The listing builds one solid part. Answer for the finished solid, in the listing's coordinates (mm). A direction names the side the tool comes from. Coordinates: 2 decimals unless noted, no trailing zeros. Write each loop counter-clockwise with the first axis right and the second up, starting at its lowest first coordinate (ties: lowest second). Pieces come first, ordered by that corner, then holes. Notation, with made-up numbers: M 55.5,37 L 101.5,37 A28 ccw 101.5,62 Z; hole C -3,43.5 d2. An arc over 180 degrees is marked long. Answer as CSV lines item,"result".
```python
from build123d import *

# Parameters (mm, degrees)
BOSS_EXTRUDE1_DEPTH = 1.57
SKETCH2_W           = 4.040944922
SKETCH2_H           = 4.040944922
BOSS_EXTRUDE2_DEPTH = 1.57


with BuildPart() as part:
    # Sketch1 → Boss-Extrude1 (new body)
    with BuildSketch(Plane.XY):
        with BuildLine():
            Line((10, 2), (10, 40))
            Line((10, 40), (0, 40))
            Line((0, 40), (0, 32))
            ThreePointArc((0, 32), (1.414213562, 31.414213562), (2, 30))
            ThreePointArc((2, 30), (1.414213562, 28.585786438), (0, 28))
            Line((0, 28), (0, 12.75))
            ThreePointArc((0, 12.75), (1.944543648, 11.944543648), (2.75, 10))
            ThreePointArc((2.75, 10), (1.944543648, 8.055456352), (0, 7.25))
            Line((0, 7.25), (0, 0))
            Line((0, 0), (8, 0))
            ThreePointArc((8, 0), (8.585786438, 1.414213562), (10, 2))
        make_face()
        with BuildLine():
            Line((20, 40), (10, 40))
            Line((10, 40), (10, 2))
            ThreePointArc((10, 2), (11.414213562, 1.414213562), (12, 0))
            Line((12, 0), (20, 0))
            Line((20, 0), (20, 7.25))
            ThreePointArc((20, 7.25), (17.25, 10), (20, 12.75))
            Line((20, 12.75), (20, 28))
            ThreePointArc((20, 28), (18, 30), (20, 32))
            Line((20, 32), (20, 40))
        make_face()
        with BuildLine():
            ThreePointArc((2, 30), (1.414213562, 31.414213562), (0, 32))
            Line((0, 32), (0, 31.11))
            ThreePointArc((0, 31.11), (0.784888527, 30.784888527), (1.11, 30))
            ThreePointArc((1.11, 30), (0.784888527, 29.215111473), (0, 28.89))
            Line((0, 28.89), (0, 28))
            ThreePointArc((0, 28), (1.414213562, 28.585786438), (2, 30))
        make_face()
        with BuildLine():
            Line((0, 31.11), (0, 32))
            ThreePointArc((0, 32), (-2, 30), (0, 28))
            Line((0, 28), (0, 28.89))
            ThreePointArc((0, 28.89), (-1.11, 30), (0, 31.11))
        make_face()
        with BuildLine():
            ThreePointArc((22, 30), (21.414213562, 31.414213562), (20, 32))
            Line((20, 32), (20, 31.11))
            ThreePointArc((20, 31.11), (20.784888527, 30.784888527), (21.11, 30))
            ThreePointArc((21.11, 30), (20.784888527, 29.215111473), (20, 28.89))
            Line((20, 28.89), (20, 28))
            ThreePointArc((20, 28), (21.414213562, 28.585786438), (22, 30))
        make_face()
        with BuildLine():
            Line((20, 31.11), (20, 32))
            ThreePointArc((20, 32), (18, 30), (20, 28))
            Line((20, 28), (20, 28.89))
            ThreePointArc((20, 28.89), (18.89, 30), (20, 31.11))
        make_face()
        with BuildLine():
            ThreePointArc((8, 0), (10, -2), (12, 0))
            Line((12, 0), (11.11, 0))
            ThreePointArc((11.11, 0), (10, -1.11), (8.89, 0))
            Line((8.89, 0), (8, 0))
        make_face()
        with BuildLine():
            ThreePointArc((12, 0), (11.414213562, 1.414213562), (10, 2))
            Line((10, 2), (10, 1.11))
            ThreePointArc((10, 1.11), (10.784888527, 0.784888527), (11.11, 0))
            Line((11.11, 0), (12, 0))
        make_face()
        with BuildLine():
            Line((10, 1.11), (10, 2))
            ThreePointArc((10, 2), (8.585786438, 1.414213562), (8, 0))
            Line((8, 0), (8.89, 0))
            ThreePointArc((8.89, 0), (9.215111473, 0.784888527), (10, 1.11))
        make_face()
    extrude(amount=BOSS_EXTRUDE1_DEPTH)

    # Sketch2 → Boss-Extrude2 (add)
    with BuildSketch(Plane(origin=(0, 0, 0), x_dir=(-1, 0, 0), z_dir=(0, 0, -1))):
        with Locations((-10, 10)):
            Rectangle(SKETCH2_W, SKETCH2_H)
    extrude(amount=BOSS_EXTRUDE2_DEPTH)


solid = part.part
```
Q1. For faces 1 (the flat face through (20, 20, 1)), 2 (the flat face through (0, 36, 1)), 3 (the flat face through (12.02, 10, -1)), 4 (the flat face through (20, 36, 1)), 5 (the flat face through (0, 20, 1)), determine the directions among +Z, -Z, +X, -X, +Y, -Y from which every point of the face is accessible in a straight line to the end or side of a thin tool.
Output:
face 1,"+Z, -Z, +X, -Y"
face 2,"+Z, -Z, -X, +Y"
face 3,"-Z, +X, +Y, -Y"
face 4,"+Z, -Z, +X, +Y"
face 5,"+Z, -Z, -X, -Y"
Q2. Find section B-B (x = 1.75). Give the vertices of the cut face in (y, z).
Output:
outline,"M 0,0 L 7.88,0 L 7.88,1.57 L 0,1.57 Z; M 12.12,0 L 40,0 L 40,1.57 L 12.12,1.57 Z"
Q3. Find section C-C (y = 16.5). Give the vertices of the cut face in (x, z), and give its area (3 significant figures).
Output:
outline,"M 0,0 L 20,0 L 20,1.57 L 0,1.57 Z"
area,"31.4 mm2"
Q4. Straight lines are drawn through the part: line 1 (X direction, y = 30, z = 0.5); line 2 (Z direction, x = 17, y = 24); line 3 (X direction, y = 25, z = 0.3). For each, find the intervals that lie inside material, in ascending order.
Output:
line 1,"-2 to -1.11, 1.11 to 18.89, 21.11 to 22"
line 2,"0 to 1.57"
line 3,"0 to 20"
Q5. Find section D-D (x = 16.5). Give the vertices of the cut face in (y, z).
Output:
outline,"M 0,0 L 40,0 L 40,1.57 L 0,1.57 Z"
Q6. Find section A-A (z = 0.8). Give the vertices of the cut face in (x, y), and give its area (3 significant figures).
Output:
outline,"M 0,0 L 8,0 A2 ccw 12,0 L 20,0 L 20,7.25 A2.75 cw 20,12.75 L 20,28 A2 ccw 20,32 L 20,40 L 0,40 L 0,32 A2 ccw 0,28 L 0,12.75 A2.75 cw 0,7.25 Z; hole C 0,30 d2.22; hole C 10,0 d2.22; hole C 20,30 d2.22"
area,"783 mm2"
Q7. Flat-ended cylindrical pins translate along their axes: pin 1 Ø0.8 at (x, z) = (9.5, -1) entering from +Y; pin 2 Ø0.8 at (y, z) = (2.5, 1) entering from +X; pin 3 Ø0.8 at (y, z) = (10.5, -0.5) entering from -X. Find the tip coordinate at first contact, or state that the pin passes through.
Output:
pin 1,"y = 12.02"
pin 2,"x = 20"
pin 3,"x = 7.98"
